Could you check a few things on this model? Use its own coordinates, in mm. Round coordinates to 2 decimals unless told otherwise and drop trailing zeros. Write each loop counter-clockwise with the first axis right and the second up, starting at its lowest first coordinate (ties: lowest second). Pieces come first, ordered by that corner, then holes. Notation, with made-up numbers: (-7.5, 74) -> (33.5, 74) arc R8 ccw to (33.5, 88) -> close; hole circle Ø9 at (14.5, 81). An arc over 180 degrees is marked (long way). Return JSON: item names as keys, results as strings.
from build123d import *

# Parameters (mm, degrees)
SKETCH1_R           = 3.175
BOSS_EXTRUDE1_DEPTH = 12.7
SKETCH2_R           = 3.175
CUT_EXTRUDE1_DEPTH  = 12.7
SKETCH3_R           = 3.3734375
CUT_EXTRUDE2_DEPTH  = 12.7
CUT_EXTRUDE3_START  = -6.35
SKETCH3_3_R         = 5.55625
SKETCH3_3_R_2       = 3.3734375
CUT_EXTRUDE3_DEPTH  = 6.35
SKETCH5_R           = 3.3734375
CUT_EXTRUDE4_DEPTH  = 12.7
SKETCH5_3_R         = 5.55625
SKETCH5_3_R_2       = 3.3734375
CUT_EXTRUDE5_DEPTH  = 6.35


with BuildPart() as part:
    # Sketch1 → Boss-Extrude1 (new body)
    with BuildSketch(Plane.XY):
        Polygon((0, 152.4), (0, 0), (63.5, 0), (63.5, 50.8), (215.9, 50.8), (215.9, -76.2), (285.75, -76.2), (285.75, 152.4), align=None)
        with Locations((19.05, 12.7)):
            Circle(SKETCH1_R, mode=Mode.SUBTRACT)
        with Locations((19.05, 38.1)):
            Circle(SKETCH1_R, mode=Mode.SUBTRACT)
        with Locations((44.45, 12.7)):
            Circle(SKETCH1_R, mode=Mode.SUBTRACT)
        with Locations((44.45, 38.1)):
            Circle(SKETCH1_R, mode=Mode.SUBTRACT)
        with Locations((247.65, 12.7)):
            Circle(SKETCH1_R, mode=Mode.SUBTRACT)
        with Locations((247.65, 38.1)):
            Circle(SKETCH1_R, mode=Mode.SUBTRACT)
        with Locations((44.45, 63.5)):
            Circle(SKETCH1_R, mode=Mode.SUBTRACT)
        with Locations((69.85, 63.5)):
            Circle(SKETCH1_R, mode=Mode.SUBTRACT)
        with Locations((44.45, 88.9)):
            Circle(SKETCH1_R, mode=Mode.SUBTRACT)
        with Locations((69.85, 88.9)):
            Circle(SKETCH1_R, mode=Mode.SUBTRACT)
        with Locations((95.25, 63.5)):
            Circle(SKETCH1_R, mode=Mode.SUBTRACT)
        with Locations((120.65, 63.5)):
            Circle(SKETCH1_R, mode=Mode.SUBTRACT)
        with Locations((95.25, 88.9)):
            Circle(SKETCH1_R, mode=Mode.SUBTRACT)
        with Locations((120.65, 88.9)):
            Circle(SKETCH1_R, mode=Mode.SUBTRACT)
        with Locations((19.05, 114.3)):
            Circle(SKETCH1_R, mode=Mode.SUBTRACT)
        with Locations((44.45, 114.3)):
            Circle(SKETCH1_R, mode=Mode.SUBTRACT)
        with Locations((69.85, 114.3)):
            Circle(SKETCH1_R, mode=Mode.SUBTRACT)
        with Locations((19.05, 139.7)):
            Circle(SKETCH1_R, mode=Mode.SUBTRACT)
        with Locations((44.45, 139.7)):
            Circle(SKETCH1_R, mode=Mode.SUBTRACT)
        with Locations((69.85, 139.7)):
            Circle(SKETCH1_R, mode=Mode.SUBTRACT)
        with Locations((95.25, 114.3)):
            Circle(SKETCH1_R, mode=Mode.SUBTRACT)
        with Locations((120.65, 114.3)):
            Circle(SKETCH1_R, mode=Mode.SUBTRACT)
        with Locations((95.25, 139.7)):
            Circle(SKETCH1_R, mode=Mode.SUBTRACT)
        with Locations((120.65, 139.7)):
            Circle(SKETCH1_R, mode=Mode.SUBTRACT)
        with Locations((146.05, 63.5)):
            Circle(SKETCH1_R, mode=Mode.SUBTRACT)
        with Locations((171.45, 63.5)):
            Circle(SKETCH1_R, mode=Mode.SUBTRACT)
        with Locations((196.85, 63.5)):
            Circle(SKETCH1_R, mode=Mode.SUBTRACT)
        with Locations((146.05, 88.9)):
            Circle(SKETCH1_R, mode=Mode.SUBTRACT)
        with Locations((171.45, 88.9)):
            Circle(SKETCH1_R, mode=Mode.SUBTRACT)
        with Locations((196.85, 88.9)):
            Circle(SKETCH1_R, mode=Mode.SUBTRACT)
        with Locations((222.25, 63.5)):
            Circle(SKETCH1_R, mode=Mode.SUBTRACT)
        with Locations((247.65, 63.5)):
            Circle(SKETCH1_R, mode=Mode.SUBTRACT)
        with Locations((273.05, 63.5)):
            Circle(SKETCH1_R, mode=Mode.SUBTRACT)
        with Locations((222.25, 88.9)):
            Circle(SKETCH1_R, mode=Mode.SUBTRACT)
        with Locations((247.65, 88.9)):
            Circle(SKETCH1_R, mode=Mode.SUBTRACT)
        with Locations((273.05, 88.9)):
            Circle(SKETCH1_R, mode=Mode.SUBTRACT)
        with Locations((146.05, 114.3)):
            Circle(SKETCH1_R, mode=Mode.SUBTRACT)
        with Locations((171.45, 114.3)):
            Circle(SKETCH1_R, mode=Mode.SUBTRACT)
        with Locations((196.85, 114.3)):
            Circle(SKETCH1_R, mode=Mode.SUBTRACT)
        with Locations((146.05, 139.7)):
            Circle(SKETCH1_R, mode=Mode.SUBTRACT)
        with Locations((171.45, 139.7)):
            Circle(SKETCH1_R, mode=Mode.SUBTRACT)
        with Locations((196.85, 139.7)):
            Circle(SKETCH1_R, mode=Mode.SUBTRACT)
        with Locations((222.25, 114.3)):
            Circle(SKETCH1_R, mode=Mode.SUBTRACT)
        with Locations((247.65, 114.3)):
            Circle(SKETCH1_R, mode=Mode.SUBTRACT)
        with Locations((273.05, 114.3)):
            Circle(SKETCH1_R, mode=Mode.SUBTRACT)
        with Locations((222.25, 139.7)):
            Circle(SKETCH1_R, mode=Mode.SUBTRACT)
        with Locations((247.65, 139.7)):
            Circle(SKETCH1_R, mode=Mode.SUBTRACT)
        with Locations((273.05, 139.7)):
            Circle(SKETCH1_R, mode=Mode.SUBTRACT)
    extrude(amount=BOSS_EXTRUDE1_DEPTH)

    # Sketch2 → Cut-Extrude1 (cut)
    with BuildSketch(Plane.XY.offset(12.7)):
        with Locations((247.65, -12.7)):
            Circle(SKETCH2_R)
        with Locations((247.65, -38.1)):
            Circle(SKETCH2_R)
        with Locations((247.65, -63.5)):
            Circle(SKETCH2_R)
        with Locations((273.05, -38.1)):
            Circle(SKETCH2_R)
        with Locations((273.05, -63.5)):
            Circle(SKETCH2_R)
        with Locations((273.05, 38.1)):
            Circle(SKETCH2_R)
    extrude(amount=-CUT_EXTRUDE1_DEPTH, mode=Mode.SUBTRACT)

    # Sketch3 → Cut-Extrude2 (cut)
    with BuildSketch(Plane.XY.offset(12.7)):
        with Locations((257.175, -3.2258)):
            Circle(SKETCH3_R)
        with Locations((257.175, 22.1742)):
            Circle(SKETCH3_R)
    extrude(amount=-CUT_EXTRUDE2_DEPTH, mode=Mode.SUBTRACT)

    # Sketch3<3> → Cut-Extrude3 (cut)
    # profile 1 of 2: a face of its own
    with BuildSketch(Plane.XY.offset(12.7).offset(CUT_EXTRUDE3_START)):
        with Locations((257.175, -3.2258)):
            Circle(SKETCH3_3_R)
        with Locations((257.175, -3.2258)):
            Circle(SKETCH3_3_R_2, mode=Mode.SUBTRACT)
    # profile 2 of 2: a face of its own
    with BuildSketch(Plane.XY.offset(12.7).offset(CUT_EXTRUDE3_START)):
        with Locations((257.175, 22.1742)):
            Circle(SKETCH3_3_R)
        with Locations((257.175, 22.1742)):
            Circle(SKETCH3_3_R_2, mode=Mode.SUBTRACT)
    extrude(amount=-CUT_EXTRUDE3_DEPTH, mode=Mode.SUBTRACT)

    # Sketch5 → Cut-Extrude4 (cut)
    with BuildSketch(Plane(origin=(0, 0, 0), x_dir=(-1, 0, 0), z_dir=(0, 0, -1))):
        with Locations((-23.114, 61.3918)):
            Circle(SKETCH5_R)
        with Locations((-23.114, 86.7918)):
            Circle(SKETCH5_R)
    extrude(amount=-CUT_EXTRUDE4_DEPTH, mode=Mode.SUBTRACT)

    # Sketch5<3> → Cut-Extrude5 (cut)
    # profile 1 of 2: a face of its own
    with BuildSketch(Plane(origin=(0, 0, 0), x_dir=(-1, 0, 0), z_dir=(0, 0, -1))):
        with Locations(Location((-23.114, 61.3918, 0), (0, 0, 180))):
            Circle(SKETCH5_3_R)
        with Locations((-23.114, 61.3918)):
            Circle(SKETCH5_3_R_2, mode=Mode.SUBTRACT)
    # profile 2 of 2: a face of its own
    with BuildSketch(Plane(origin=(0, 0, 0), x_dir=(-1, 0, 0), z_dir=(0, 0, -1))):
        with Locations(Location((-23.114, 86.7918, 0), (0, 0, 180))):
            Circle(SKETCH5_3_R)
        with Locations((-23.114, 86.7918)):
            Circle(SKETCH5_3_R_2, mode=Mode.SUBTRACT)
    extrude(amount=-CUT_EXTRUDE5_DEPTH, mode=Mode.SUBTRACT)


solid = part.part
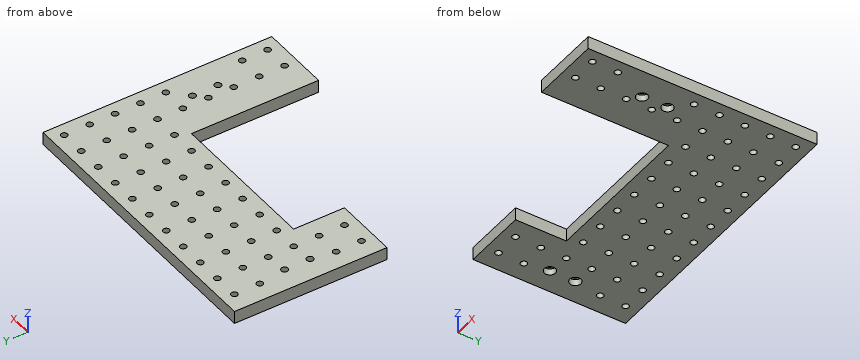
1) I want a section at C-C, the plane x = 222.25. Please give me the cut outline in (y, z) (3 decimals).
Return value:
{"outline": "(-76.2, 0) -> (60.325, 0) -> (60.325, 12.7) -> (-76.2, 12.7) -> close; (66.675, 0) -> (85.725, 0) -> (85.725, 12.7) -> (66.675, 12.7) -> close; (92.075, 0) -> (111.125, 0) -> (111.125, 12.7) -> (92.075, 12.7) -> close; (117.475, 0) -> (136.525, 0) -> (136.525, 12.7) -> (117.475, 12.7) -> close; (142.875, 0) -> (152.4, 0) -> (152.4, 12.7) -> (142.875, 12.7) -> close"}
2) Will these pins go through, and if not, where does the flat tip stop? pin 1 Ø6 at (y, z) = (-40.5, 8) entering from -X; pin 2 Ø1.5 at (x, z) = (150, 6) entering from -Y; pin 3 Ø4 at (x, z) = (53.5, 9.5) entering from -Y.
Return value:
{"pin 1": "x = 215.9", "pin 2": "y = 50.8", "pin 3": "y = 0"}
3) I want a section at B-B, the plane y = 114.3. Count the separate pieces of the cut face and the enclosed holes in it, and give its area (3 significant figures).
Return value:
{"separate pieces": "12", "enclosed holes": "0", "area": "2,740 mm²"}
4) I want a section at A-A, the plane x = 69.85. Please give me the cut outline in (y, z) (3 decimals), and give its area (3 significant figures).
Return value:
{"outline": "(50.8, 0) -> (60.325, 0) -> (60.325, 12.7) -> (50.8, 12.7) -> close; (66.675, 0) -> (85.725, 0) -> (85.725, 12.7) -> (66.675, 12.7) -> close; (92.075, 0) -> (111.125, 0) -> (111.125, 12.7) -> (92.075, 12.7) -> close; (117.475, 0) -> (136.525, 0) -> (136.525, 12.7) -> (117.475, 12.7) -> close; (142.875, 0) -> (152.4, 0) -> (152.4, 12.7) -> (142.875, 12.7) -> close", "area": "968 mm²"}
5) If I drill on probe 1 along Y at (x, z) = (69.85, 3) (3 decimals); probe 2 along Y at (x, z) = (19.5, 7); probe 3 along X at (y, z) = (17, 9), over which ranges is the centre line in solid material (lowest first)? Write a range as [from, to].
Return value:
{"probe 1": "[50.8, 60.325], [66.675, 85.725], [92.075, 111.125], [117.475, 136.525], [142.875, 152.4]", "probe 2": "[0, 9.56], [15.84, 34.96], [41.24, 111.16], [117.44, 136.56], [142.84, 152.4]", "probe 3": "[0, 63.5], [215.9, 285.75]"}
